from build123d import *

# Parameters (mm, degrees)
F0_R     = 11.2
F1_DEPTH = 7
F2_DEPTH = 7


with BuildPart() as f1:
    # F0 (on Top) → F1 (new body)
    with BuildSketch(Plane.XY):
        with BuildLine():
            ThreePointArc((9.814137, 6.603833), (7.749518, 11.690361), (9.702716, 16.820705))
            ThreePointArc((9.702716, 16.820705), (0, 43.259993), (-9.702716, 16.820705))
            ThreePointArc((-9.702716, 16.820705), (-7.749518, 11.690361), (-9.814137, 6.603833))
            ThreePointArc((-9.814137, 6.603833), (-12.998756, 2.745467), (-14.737406, -1.945575))
            ThreePointArc((-14.737406, -1.945575), (-13.075563, -12.090494), (-5.272209, -18.782935))
            ThreePointArc((-5.272209, -18.782935), (-0.239573, -19.738094), (4.821001, -18.94416))
            ThreePointArc((4.821001, -18.94416), (12.802187, -12.556912), (14.837681, -2.539276))
            ThreePointArc((14.837681, -2.539276), (13.146374, 2.483071), (9.814137, 6.603833))
        make_face()
        with Locations((0, -4.740007)):
            Circle(F0_R, mode=Mode.SUBTRACT)
        with Locations((0, 28.259993)):
            Circle(F0_R, mode=Mode.SUBTRACT)
    extrude(amount=F1_DEPTH)

    # F0 (on Top) → F2 (join)
    with BuildSketch(Plane.XY):
        with BuildLine():
            ThreePointArc((9.814137, 6.603833), (7.749518, 11.690361), (9.702716, 16.820705))
            ThreePointArc((9.702716, 16.820705), (0, 43.259993), (-9.702716, 16.820705))
            ThreePointArc((-9.702716, 16.820705), (-7.749518, 11.690361), (-9.814137, 6.603833))
            ThreePointArc((-9.814137, 6.603833), (-12.998756, 2.745467), (-14.737406, -1.945575))
            ThreePointArc((-14.737406, -1.945575), (-13.075563, -12.090494), (-5.272209, -18.782935))
            ThreePointArc((-5.272209, -18.782935), (-0.239573, -19.738094), (4.821001, -18.94416))
            ThreePointArc((4.821001, -18.94416), (12.802187, -12.556912), (14.837681, -2.539276))
            ThreePointArc((14.837681, -2.539276), (13.146374, 2.483071), (9.814137, 6.603833))
        make_face()
        with Locations((0, -4.740007)):
            Circle(F0_R, mode=Mode.SUBTRACT)
        with Locations((0, 28.259993)):
            Circle(F0_R, mode=Mode.SUBTRACT)
        with BuildLine():
            ThreePointArc((23.427499, -7.150505), (18.281136, -6.430983), (14.837681, -2.539276))
            ThreePointArc((14.837681, -2.539276), (12.802187, -12.556912), (4.821001, -18.94416))
            ThreePointArc((4.821001, -18.94416), (10.258373, -19.699411), (13.724783, -23.956102))
            ThreePointArc((13.724783, -23.956102), (41.473236, -28.772947), (23.427499, -7.150505))
        make_face()
        with Locations((28.482855, -21.272947)):
            Circle(F0_R, mode=Mode.SUBTRACT)
        with BuildLine():
            ThreePointArc((-5.272209, -18.782935), (-13.075563, -12.090494), (-14.737406, -1.945575))
            ThreePointArc((-14.737406, -1.945575), (-18.16346, -6.243294), (-23.600001, -7.050911))
            ThreePointArc((-23.600001, -7.050911), (-41.645738, -28.673353), (-13.897285, -23.856507))
            ThreePointArc((-13.897285, -23.856507), (-10.554578, -19.671007), (-5.272209, -18.782935))
        make_face()
        with Locations((-28.655357, -21.173353)):
            Circle(F0_R, mode=Mode.SUBTRACT)
    extrude(amount=F2_DEPTH)


solid = f1.part
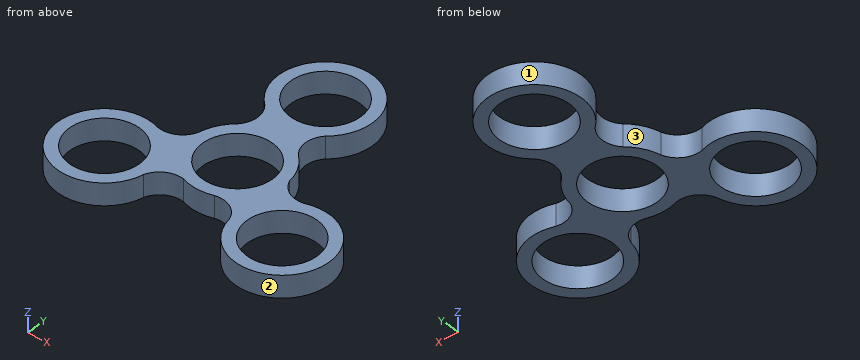
Geometry: final body of the model. Coordinates: model frame, mm. Face numbers are marked on the shaded views. Give positions to 0.01 mm unless a question says otherwise; leave off trailing zeros. Write each loop counter-clockwise with the first axis right and the second up, starting at its lowest first coordinate (ties: lowest second). Pieces come first, ordered by that corner, then holes. Notation, with made-up numbers: M 78,-32 L 91,-32 A37 ccw 91,4 Z; hole C -40,18.5 d6. An arc over 180 degrees is marked long. Answer in a Markdown table with one row per item. Add a question column.
(1) Mould query, pull axis X, two halves, no side actions, for the marked faces 1, 2 and 3. Classes: +X half, -X half, draft (parallel to the pull), parting line (faces both ways), or undercut.
(2) Section B-B on y = -25. Return loops of the section in (x, z), and give its area (3 significant figures).
(3) Section A-A on x = 0. Return loops of the section in (y, z), and give its area (3 significant figures).
(4) Section C-C on x = -25. Return loops of the section in (y, z).
(5) Section D-D on y = 25. Return loops of the section in (x, z), and give its area (3 significant figures).
(6) First-contact query: pin 1 (3 mm diameter, centred on y = 19, z = 4, fed in from +X); pin 2 (4 mm diameter, centred on x = 14, z = 2, fed in from +Y); pin 3 (1.5 mm diameter, centred on x = -14, z = 6, fed in from -Y). Flat tips, straight axial feed; report the tip coordinate or a pass-through.
(7) Ray query, line 1 (Y direction, x = 0, z = 3); line 2 (X direction, y = -12.5, z = 2.75); line 3 (Y direction, x = -3, z = 5). Return the intervals inside material, ascending.
Result set:
| question | item | result |
|---|---|---|
| 1 | face 1 | parting line |
| 1 | face 2 | undercut |
| 1 | face 3 | -X half |
| 2 | outline | M -43.16,0 L -39.18,0 L -39.18,7 L -43.16,7 Z; M -18.13,0 L -14.15,0 L -14.15,7 L -18.13,7 Z; M 13.95,0 L 17.92,0 L 17.92,7 L 13.95,7 Z; M 39.04,0 L 43.01,0 L 43.01,7 L 39.04,7 Z |
| 2 | area | 111 mm^2 |
| 3 | outline | M -19.74,0 L -15.94,0 L -15.94,7 L -19.74,7 Z; M 6.46,0 L 17.06,0 L 17.06,7 L 6.46,7 Z; M 39.46,0 L 43.26,0 L 43.26,7 L 39.46,7 Z |
| 3 | area | 127 mm^2 |
| 4 | outline | M -35.72,0 L -31.76,0 L -31.76,7 L -35.72,7 Z; M -10.59,0 L -6.63,0 L -6.63,7 L -10.59,7 Z |
| 5 | outline | M -14.64,0 L -10.72,0 L -10.72,7 L -14.64,7 Z; M 10.72,0 L 14.64,0 L 14.64,7 L 10.72,7 Z |
| 5 | area | 55.0 mm^2 |
| 6 | pin 1 | stops at x = 12.84 |
| 6 | pin 2 | stops at y = 37.26 |
| 6 | pin 3 | stops at y = -26.8 |
| 7 | line 1 | y = -19.74 to -15.94, 6.46 to 17.06, 39.46 to 43.26 |
| 7 | line 2 | x = -40.89 to -35.74, -21.57 to -8.08, 8.08 to 21.52, 35.45 to 40.65 |
| 7 | line 3 | y = -19.44 to -15.53, 6.05 to 17.47, 39.05 to 42.96 |
